Read the model definition and answer for the solid it produces. Units are mm, in the model's axes. Coordinates: 2 decimals unless noted, no trailing zeros. Loops run counter-clockwise (first coordinate to the right, second up) from the corner with the lowest first, then second, coordinate; pieces in that order, holes last. Notation, with made-up numbers: M 70,75 L 92,75 A11 ccw 92,95 Z; hole C -38,87.5 d4. An arc over 180 degrees is marked long. Put each result on its own line as item: value.
from build123d import *

# Parameters (mm, degrees)
SKETCH1_W                      = 203.2
SKETCH1_H                      = 60
SKETCH1_R                      = 3.3
SKETCH1_R_2                    = 3.5
BOSS_EXTRUDE1_DEPTH            = 3.175
SKETCH2_R                      = 3.2639
F_1_4_20_FOR_NUT_BRACKET_DEPTH = 106.984152707
SKETCH3_R                      = 0.79375
SKETCH3_R_2                    = 1.27
WIRE_HOLDER_DEPTH              = 106.984152707
SKETCH4_R                      = 3.3
CUT_EXTRUDE1_DEPTH             = 106.984152707


with BuildPart() as part:
    # Sketch1 → Boss-Extrude1 (new body)
    with BuildSketch(Plane(origin=(0, 0, 0), x_dir=(1, 0, 0), z_dir=(0, 1, 0))):
        Rectangle(SKETCH1_W, SKETCH1_H)
        with Locations(Location((-52.4, 20, 0), (0, 0, 270))):
            Circle(SKETCH1_R, mode=Mode.SUBTRACT)
        with Locations(Location((-92.4, -20, 0), (0, 0, 90))):
            Circle(SKETCH1_R_2, mode=Mode.SUBTRACT)
        with Locations(Location((-52.4, -20, 0), (0, 0, 90))):
            Circle(SKETCH1_R, mode=Mode.SUBTRACT)
        with Locations(Location((92.4, 20, 0), (0, 0, 90))):
            Circle(SKETCH1_R_2, mode=Mode.SUBTRACT)
        with Locations(Location((-92.4, 20, 0), (0, 0, 270))):
            Circle(SKETCH1_R_2, mode=Mode.SUBTRACT)
        with Locations(Location((52.4, -20, 0), (0, 0, 270))):
            Circle(SKETCH1_R, mode=Mode.SUBTRACT)
        with Locations(Location((92.4, -20, 0), (0, 0, 270))):
            Circle(SKETCH1_R_2, mode=Mode.SUBTRACT)
        with Locations(Location((52.4, 20, 0), (0, 0, 90))):
            Circle(SKETCH1_R, mode=Mode.SUBTRACT)
    extrude(amount=BOSS_EXTRUDE1_DEPTH)

    # Sketch2 → 1/4-20 for Nut Bracket (cut, through all)
    with BuildSketch(Plane(origin=(0, 3.175, 0), x_dir=(1, 0, 0), z_dir=(0, 1, 0))):
        with Locations(Location((-12.7, -17.3, 0), (0, 0, 270))):
            Circle(SKETCH2_R)
        with Locations(Location((12.7, -17.3, 0), (0, 0, 270))):
            Circle(SKETCH2_R)
        with Locations(Location((0, 0.48, 0), (0, 0, 270))):
            Circle(SKETCH2_R)
    extrude(amount=-F_1_4_20_FOR_NUT_BRACKET_DEPTH, mode=Mode.SUBTRACT)

    # Sketch3 → Wire Holder (cut, through all)
    with BuildSketch(Plane(origin=(0, 3.175, 0), x_dir=(1, 0, 0), z_dir=(0, 1, 0))):
        with Locations(Location((-31.6, -15, 0), (0, 0, 270))):
            Circle(SKETCH3_R)
        with Locations(Location((-31.6, -8.65, 0), (0, 0, 270))):
            Circle(SKETCH3_R_2)
        with Locations(Location((-31.6, -21.35, 0), (0, 0, 270))):
            Circle(SKETCH3_R_2)
    extrude(amount=-WIRE_HOLDER_DEPTH, mode=Mode.SUBTRACT)

    # Sketch4 → Cut-Extrude1 (cut, through all)
    with BuildSketch(Plane(origin=(0, 3.175, 0), x_dir=(1, 0, 0), z_dir=(0, 1, 0))):
        with Locations(Location((28.9, -20, 0), (0, 0, 270))):
            Circle(SKETCH4_R)
        with Locations(Location((28.9, 20, 0), (0, 0, 270))):
            Circle(SKETCH4_R)
    extrude(amount=-CUT_EXTRUDE1_DEPTH, mode=Mode.SUBTRACT)


solid = part.part
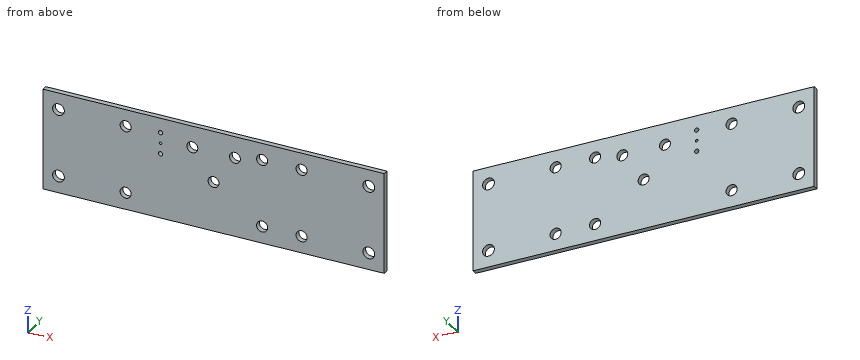
1) Find section A-A, the plane x = -92.4. Write down the section's boundary in (y, z) (3 decimals), plus the area to 3 significant figures.
Answer list:
outline: M 0,-30 L 3.175,-30 L 3.175,-23.5 L 0,-23.5 Z; M 0,-16.5 L 3.175,-16.5 L 3.175,16.5 L 0,16.5 Z; M 0,23.5 L 3.175,23.5 L 3.175,30 L 0,30 Z
area: 146 mm^2
2) Find section C-C, the plane z = -0.48. Write down the section's boundary in (x, y) (3 decimals), plus the area to 3 significant figures.
Answer list:
outline: M -101.6,0 L -3.264,0 L -3.264,3.175 L -101.6,3.175 Z; M 3.264,0 L 101.6,0 L 101.6,3.175 L 3.264,3.175 Z
area: 624 mm^2
3) Find section B-B, the plane y = 1.9. Count the separate pieces of the cut face and the enclosed holes in it, plus the area to 3 significant figures.
Answer list:
separate pieces: 1
enclosed holes: 16
area: 11,700 mm^2
4) Straight lines are drawn through the part: line 1 (X direction, y = 1.45, z = -20); line 2 (X direction, y = 1.2, z = -22); line 3 (X direction, y = 0.8, z = -0.48). For each, find the intervals that lie inside material, in ascending order. Write a range as [from, to].
Answer list:
line 1: x = [-101.6, -95.9], [-88.9, -55.7], [-49.1, 25.6], [32.2, 49.1], [55.7, 88.9], [95.9, 101.6]
line 2: x = [-101.6, -95.27], [-89.53, -55.02], [-49.78, 26.28], [31.52, 49.78], [55.02, 89.53], [95.27, 101.6]
line 3: x = [-101.6, -3.26], [3.26, 101.6]
5) Find section D-D, the plane z = -19.5. Write down the section's boundary in (x, y) (3 decimals).
Answer list:
outline: M -101.6,0 L -95.864,0 L -95.864,3.175 L -101.6,3.175 Z; M -88.936,0 L -55.662,0 L -55.662,3.175 L -88.936,3.175 Z; M -49.138,0 L 25.638,0 L 25.638,3.175 L -49.138,3.175 Z; M 32.162,0 L 49.138,0 L 49.138,3.175 L 32.162,3.175 Z; M 55.662,0 L 88.936,0 L 88.936,3.175 L 55.662,3.175 Z; M 95.864,0 L 101.6,0 L 101.6,3.175 L 95.864,3.175 Z
